Geometry check sheet. Reference: the model listing, model coordinates, mm. Face numbers are marked on the shaded views. A direction names the side the tool comes from. Coordinates: 2 decimals unless noted, no trailing zeros. Loops run counter-clockwise (first coordinate to the right, second up) from the corner with the lowest first, then second, coordinate; pieces in that order, holes last. Notation, with made-up numbers: (-19.5, -37.75) - (3.5, -37.75) arc R12 cw to (3.5, -26.75) - close; hole circle Ø9 at (71.25, 86.25). An arc over 180 degrees is marked (long way). Write item = value, one per line. Start each with the question number.
from build123d import *

# Parameters (mm, degrees)
EXTRUDE_1_DEPTH = 5
M4X0_7_1_D      = 3.3


with BuildPart() as part:
    # ｽｹｯﾁ2 → 押し出し1 (new body, symmetric)
    with BuildSketch(Plane.XY):
        with BuildLine():
            Line((2.89985476, -0.30000001), (2.89985476, -0.39999919))
            ThreePointArc((2.89985476, -0.39999919), (3.017012051, -0.68284191), (3.29985477, -0.7999992))
            Line((3.29985477, -0.7999992), (4.799856544, -0.7999992))
            ThreePointArc((4.799856544, -0.7999992), (4.942617804, -0.859930564), (4.999820293, -1.003806973))
            ThreePointArc((4.999820293, -1.003806973), (4.950834117, -1.294473494), (4.819233264, -1.558230745))
            Line((4.819233264, -1.558230745), (3.577430107, -3.332233905))
            ThreePointArc((3.577430107, -3.332233905), (2.934071419, -3.896562924), (2.102813019, -4.100001158))
            Line((2.102813019, -4.100001158), (-2.102813019, -4.100001158))
            ThreePointArc((-2.102813019, -4.100001158), (-2.934071419, -3.896562924), (-3.577430107, -3.332233905))
            Line((-3.577430107, -3.332233905), (-4.819233264, -1.558230745))
            ThreePointArc((-4.819233264, -1.558230745), (-4.950834117, -1.294473494), (-4.999820293, -1.003806973))
            ThreePointArc((-4.999820293, -1.003806973), (-4.942617804, -0.859930564), (-4.799856544, -0.7999992))
            Line((-4.799856544, -0.7999992), (-3.29985477, -0.7999992))
            ThreePointArc((-3.29985477, -0.7999992), (-3.017012051, -0.68284191), (-2.89985476, -0.39999919))
            Line((-2.89985476, -0.39999919), (-2.89985476, -0.30000001))
            ThreePointArc((-2.89985476, -0.30000001), (-2.811986792, -0.087867969), (-2.59985475, 0))
            Line((-2.59985475, 0), (2.59985475, 0))
            ThreePointArc((2.59985475, 0), (2.811986792, -0.087867969), (2.89985476, -0.30000001))
        make_face()
    extrude(amount=EXTRUDE_1_DEPTH, both=True)

    # M4x0.7 ねじ穴1 (through all)
    with Locations(Plane(origin=(0, 0, 0), x_dir=(-1, 0, 0), z_dir=(0, 1, 0))):
        with Locations((0, 0)):
            Hole(M4X0_7_1_D / 2)


solid = part.part
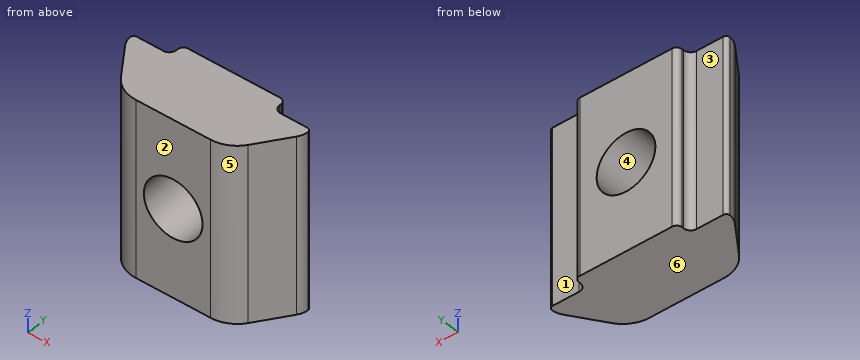
(1) Sectioned sample at A-A on x = 0. Enter the section's corners in (y, z).
(2) Sectioned sample at D-D on z = 4. Enter the section's corners in (x, y).
(3) Depth check by flat-ended pin: pin 1 (1.2 mm diameter, centred on x = -4, z = 0.5, fed in from +Y); pin 2 (1 mm diameter, centred on x = -3.5, z = 1, fed in from -Y); pin 3 (1.5 mm diameter, centred on y = -2, z = 2.5, fed in from -X). Enter the tip coordinate at first touch or a pass-through.
(4) Scan lines: line 1 (Z direction, x = 0, y = -2.05); line 2 (X direction, y = -3.3, z = -0.25); line 3 (X direction, y = -2.15, z = -1.5) (3 decimals). Record each from-to range of solid material in increasing order.
(5) Sectioned sample at B-B on z = 0. Enter the section's corners in (x, y), plus the area to 3 significant figures.
(6) Sectioned sample at C-C on y = -3. Enter the section's corners in (x, z), plus the area to 3 significant figures.
(7) Draft check along X on the marked faces 4, 5 and 6. Enter one of: pulls with the +X half, pulls with the -X half, needs draft (parallel to the pull), parting line crosses it, or undercut.
(8) Tool access check on the marked faces 1, 2 and 3. Record the directions out of +Z, -Z, +X, -X, +Y, -Y that give a thin tool (end or side, any length) a straight path to the whole face; none if there is none.
Working result:
q1.outline = (-4.1, -5) - (0, -5) - (0, -1.65) - (-4.1, -1.65) - close; (-4.1, 1.65) - (0, 1.65) - (0, 5) - (-4.1, 5) - close
q2.outline = (-5, -1) arc R1 ccw to (-4.82, -1.56) - (-3.58, -3.33) arc R1.8 ccw to (-2.1, -4.1) - (2.1, -4.1) arc R1.8 ccw to (3.58, -3.33) - (4.82, -1.56) arc R1 ccw to (5, -1) arc R0.2 ccw to (4.8, -0.8) - (3.3, -0.8) arc R0.4 cw to (2.9, -0.4) - (2.9, -0.3) arc R0.3 ccw to (2.6, 0) - (-2.6, 0) arc R0.3 ccw to (-2.9, -0.3) - (-2.9, -0.4) arc R0.4 cw to (-3.3, -0.8) - (-4.8, -0.8) arc R0.2 ccw to start
q3.pin_1 = -0.8
q3.pin_2 = -3.86
q3.pin_3 = -4.96
q4.line_1 = -5 to -1.65, 1.65 to 5
q4.line_2 = -3.6 to -1.63, 1.63 to 3.6
q4.line_3 = -4.405 to -0.687, 0.687 to 4.405
q5.outline = (-5, -1) arc R1 ccw to (-4.82, -1.56) - (-3.58, -3.33) arc R1.8 ccw to (-2.1, -4.1) - (-1.65, -4.1) - (-1.65, 0) - (-2.6, 0) arc R0.3 ccw to (-2.9, -0.3) - (-2.9, -0.4) arc R0.4 cw to (-3.3, -0.8) - (-4.8, -0.8) arc R0.2 ccw to start; (1.65, -4.1) - (2.1, -4.1) arc R1.8 ccw to (3.58, -3.33) - (4.82, -1.56) arc R1 ccw to (5, -1) arc R0.2 ccw to (4.8, -0.8) - (3.3, -0.8) arc R0.4 cw to (2.9, -0.4) - (2.9, -0.3) arc R0.3 ccw to (2.6, 0) - (1.65, 0) - close
q5.area = 18.4 mm2
q6.outline = (-3.81, -5) - (3.81, -5) - (3.81, 5) - (-3.81, 5) - close; hole circle Ø3.3 at (0, 0)
q6.area = 67.6 mm2
q7.face_4 = undercut
q7.face_5 = pulls with the +X half
q7.face_6 = needs draft
q8.face_1 = +Z, -Z, +X, +Y
q8.face_2 = +Z, -Z, +X, -X, -Y
q8.face_3 = +Z, -Z, -X, +Y
